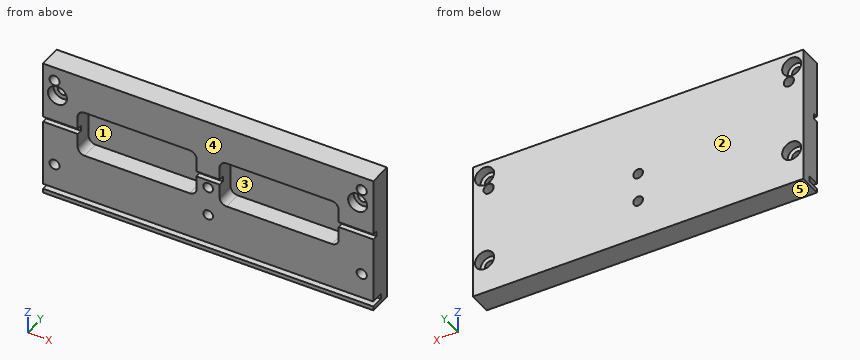
```python
from build123d import *

# Parameters (mm, degrees)
F0_W            = 143
F0_H            = 60
F1_DEPTH        = 10
F2_W            = 51.5
F2_H            = 20
F3_DEPTH        = 8
F4_R            = 3
F5_W            = 143
F5_H            = 2.3
F6_DEPTH        = 5.5
F7_W            = 143
F7_H            = 2.3
F8_DEPTH        = 2.3
F10_D           = 4.4
F10_CBORE_D     = 8.25
F10_CBORE_DEPTH = 4
F12_D           = 4.4
F12_CBORE_D     = 8.25
F12_CBORE_DEPTH = 4
F14_D           = 4.2


with BuildPart() as f1:
    # F0 (on Front) → F1 (new body)
    with BuildSketch(Plane.XZ):
        Rectangle(F0_W, F0_H)
    extrude(amount=F1_DEPTH)

    # F2 (on face) → F3 (cut)
    with BuildSketch(Plane.XZ.offset(10)):
        with Locations((-30.75, 4)):
            Rectangle(F2_W, F2_H)
        with Locations((30.75, 4)):
            Rectangle(F2_W, F2_H)
    extrude(amount=-F3_DEPTH, mode=Mode.SUBTRACT)

    # F4
    f4_edges = [f1.edges().sort_by_distance(p)[0] for p in [
        (-56.5, -6, 14),
        (-5, -6, -6),
        (56.5, -6, -6),
        (-5, -6, 14),
        (56.5, -6, 14),
        (-56.5, -6, -6),
        (5, -6, -6),
        (5, -6, 14),
    ]]
    fillet(f4_edges, radius=F4_R)

    # F5 (on face) → F6 (cut)
    with BuildSketch(Plane.XZ.offset(10)):
        with Locations((0, -27.05)):
            Rectangle(F5_W, F5_H)
    extrude(amount=-F6_DEPTH, mode=Mode.SUBTRACT)

    # F7 (on face) → F8 (cut)
    with BuildSketch(Plane.XZ.offset(10)):
        with Locations((0, 4.15)):
            Rectangle(F7_W, F7_H)
    extrude(amount=-F8_DEPTH, mode=Mode.SUBTRACT)

    # F10 (through all)
    with Locations(Plane(origin=(0, 0, 0), x_dir=(-1, 0, 0), z_dir=(0, 1, 0))):
        with Locations((-66.5, 24), (-66.5, -15), (66.5, -15), (66.5, 24)):
            CounterBoreHole(F10_D / 2, F10_CBORE_D / 2, F10_CBORE_DEPTH)

    # F12 (through all)
    with Locations(Plane.XZ.offset(10)):
        with Locations((-65.267855823, 17.5), (64.732144177, 17.5)):
            CounterBoreHole(F12_D / 2, F12_CBORE_D / 2, F12_CBORE_DEPTH)

    # F14 (through all)
    with Locations(Plane(origin=(0, 0, 0), x_dir=(-1, 0, 0), z_dir=(0, 1, 0))):
        with Locations((0, -0.3), (0, -13)):
            Hole(F14_D / 2)


solid = f1.part
```
The model under review builds one solid part; all positions refer to its coordinate system, in mm. Face numbers are marked on the shaded views. A direction names the side the tool comes from. Round coordinates to 2 decimals unless told otherwise and drop trailing zeros. Loops run counter-clockwise (first coordinate to the right, second up) from the corner with the lowest first, then second, coordinate; pieces in that order, holes last. Notation, with made-up numbers: (48, 78) -> (60, 78) arc R26 ccw to (60, 93) -> close; hole circle Ø10 at (-20.75, 47.5). An arc over 180 degrees is marked (long way). Answer in a Markdown table with one row per item.
1) Tool access review of the marked faces 1 and 2: name each direction out of +Z, -Z, +X, -X, +Y, -Y from which nothing blocks a thin tool from reaching the whole face with its end or side.
Taken from the geometry:
| item | result |
|---|---|
| face 1 | -Y |
| face 2 | +Z, -Z, +X, -X, +Y |
2) Consider section C-C, the plane x = -43.5. Write out the cut boundary in (y, z), plus the area to 3 significant figures.
Taken from the geometry:
| item | result |
|---|---|
| outline | (-10, -30) -> (0, -30) -> (0, 30) -> (-10, 30) -> (-10, 14) -> (-2, 14) -> (-2, -6) -> (-10, -6) -> (-10, -25.9) -> (-4.5, -25.9) -> (-4.5, -28.2) -> (-10, -28.2) -> close |
| area | 427 mm² |
3) Consider section B-B, the plane x = 0. Write out the cut boundary in (y, z).
Taken from the geometry:
| item | result |
|---|---|
| outline | (-10, -30) -> (0, -30) -> (0, -15.1) -> (-10, -15.1) -> (-10, -25.9) -> (-4.5, -25.9) -> (-4.5, -28.2) -> (-10, -28.2) -> close; (-10, -10.9) -> (0, -10.9) -> (0, -2.4) -> (-10, -2.4) -> close; (-10, 1.8) -> (0, 1.8) -> (0, 30) -> (-10, 30) -> (-10, 5.3) -> (-7.7, 5.3) -> (-7.7, 3) -> (-10, 3) -> close |
4) Consider section A-A, the plane z = 17.5. Write out the cut boundary in (x, y), plus the area to 3 significant figures.
Taken from the geometry:
| item | result |
|---|---|
| outline | (-71.5, -10) -> (-69.39, -10) -> (-69.39, -6) -> (-67.47, -6) -> (-67.47, 0) -> (-71.5, 0) -> close; (-63.07, -6) -> (-61.14, -6) -> (-61.14, -10) -> (60.61, -10) -> (60.61, -6) -> (62.53, -6) -> (62.53, 0) -> (-63.07, 0) -> close; (66.93, -6) -> (68.86, -6) -> (68.86, -10) -> (71.5, -10) -> (71.5, 0) -> (66.93, 0) -> close |
| area | 1,310 mm² |
5) Wall thickness on line 1 along X through (y, z) = (-5, 9.5); line 2 along Z through (x, y) = (23.5, -8.5); line 3 along Z through (x, y) = (-66.5, -5.8): over which ranges is each line inside the solid? List them lowest first.
Taken from the geometry:
| item | result |
|---|---|
| line 1 | x = -71.5 to -56.5, -5 to 5, 56.5 to 71.5 |
| line 2 | z = -30 to -28.2, -25.9 to -6, 14 to 30 |
| line 3 | z = -30 to -28.2, -25.9 to -17.2, -12.8 to 15.68, 19.32 to 21.8, 26.2 to 30 |
6) For pin 1 Ø4 at (x, z) = (0, -0.3) entering from -Y; pin 2 Ø10 at (x, z) = (-35, 7.5) entering from -Y, all flat-tipped, find the tip position at first contact; note any pin that passes through.
Taken from the geometry:
| item | result |
|---|---|
| pin 1 | passes through |
| pin 2 | stops at y = -2 |
7) Draft analysis for pull direction Z (two halves, no side actions). For the marked faces 3, 4 and 5, state which applies: pulls with the +Z half, pulls with the -Z half, needs draft (parallel to the pull), parting line crosses it, or undercut.
Taken from the geometry:
| item | result |
|---|---|
| face 3 | undercut |
| face 4 | needs draft |
| face 5 | pulls with the -Z half |
